```python
from build123d import *

# Parameters (mm, degrees)
SKETCH1_W           = 165.1
SKETCH1_H           = 76.2
SKETCH1_R           = 6.35
SKETCH1_R_2         = 2.50825
BOSS_EXTRUDE1_DEPTH = 6.35
CUT_EXTRUDE1_DEPTH  = 6.35
FILLET1_R           = 6.35
SKETCH3_R           = 1.778
CUT_EXTRUDE2_DEPTH  = 6.35
CIRPATTERN1_COUNT   = 8


with BuildPart() as part:
    # Sketch1 → Boss-Extrude1 (new body)
    with BuildSketch(Plane.XY):
        Rectangle(SKETCH1_W, SKETCH1_H)
        with Locations((0, -19.05)):
            Circle(SKETCH1_R, mode=Mode.SUBTRACT)
        with Locations((-75.40625, 31.75)):
            Circle(SKETCH1_R_2, mode=Mode.SUBTRACT)
        with Locations((75.40625, 31.75)):
            Circle(SKETCH1_R_2, mode=Mode.SUBTRACT)
        with Locations((75.40625, 19.05)):
            Circle(SKETCH1_R_2, mode=Mode.SUBTRACT)
        with Locations((-75.40625, 19.05)):
            Circle(SKETCH1_R_2, mode=Mode.SUBTRACT)
    extrude(amount=BOSS_EXTRUDE1_DEPTH)

    # Sketch2 → Cut-Extrude1 (cut)
    with BuildSketch(Plane(origin=(0, 0, 0), x_dir=(-1, 0, 0), z_dir=(0, 0, -1))):
        Polygon((12.7, -38.1), (82.55, 12.7), (82.55, -38.1), align=None)
        Polygon((-82.55, -38.1), (-82.55, 12.7), (-12.7, -38.1), align=None)
    extrude(amount=-CUT_EXTRUDE1_DEPTH, mode=Mode.SUBTRACT)

    # Fillet1
    fillet1_edges = [part.edges().sort_by_distance(p)[0] for p in [
        (-12.7, -38.1, 3.175),
        (-82.55, 12.7, 3.175),
        (12.7, -38.1, 3.175),
        (82.55, 12.7, 3.175),
        (-82.55, 38.1, 3.175),
        (82.55, 38.1, 3.175),
    ]]
    fillet(fillet1_edges, radius=FILLET1_R)

    # Sketch3 → Cut-Extrude2 (cut)
    with BuildSketch(Plane(origin=(0, 0, 0), x_dir=(-1, 0, 0), z_dir=(0, 0, -1))):
        with Locations((0, -9.271)):
            Circle(SKETCH3_R)
    cut_extrude2 = extrude(amount=-CUT_EXTRUDE2_DEPTH, mode=Mode.SUBTRACT)

    # CirPattern1: Cut-Extrude2 ×8 about axis
    cirpattern1_axis = Axis((0, -19.05, 0), (0, 0, 1))
    for i in range(1, CIRPATTERN1_COUNT):
        add(cut_extrude2.rotate(cirpattern1_axis, i * 360 / CIRPATTERN1_COUNT), mode=Mode.SUBTRACT)


solid = part.part
```
Verification items for the finished model (mm, model axes). Give positions to 0.01 mm unless a question says otherwise; leave off trailing zeros. Write each loop counter-clockwise with the first axis right and the second up, starting at its lowest first coordinate (ties: lowest second). Pieces come first, ordered by that corner, then holes. Notation, with made-up numbers: (20, 50.5) - (27, 50.5) arc R34 ccw to (27, 84.5) - close; hole circle Ø7 at (80, -38). An arc over 180 degrees is marked (long way). Put each result on its own line as item: value.
Q1. Section check A-A on x = 0. Record the cut outline in (y, z), and give its area (3 significant figures).
Result:
outline: (-38.1, 0) - (-30.61, 0) - (-30.61, 6.35) - (-38.1, 6.35) - close; (-27.05, 0) - (-25.4, 0) - (-25.4, 6.35) - (-27.05, 6.35) - close; (-12.7, 0) - (-11.05, 0) - (-11.05, 6.35) - (-12.7, 6.35) - close; (-7.49, 0) - (38.1, 0) - (38.1, 6.35) - (-7.49, 6.35) - close
area: 358 mm2
Q2. Mould release check, pull along Y, two halves, no side actions. Record for faces 1 (the face through (-1.38, -25.25, 3.13)), 2 (the face through (0, -38.1, 3)), 3 (the face through (-1, 9, 0)): released by +Y, released by -Y, zero draft, split by the parting line, or undercut.
Result:
face 1: undercut
face 2: released by -Y
face 3: zero draft
Q3. Depth check by flat-ended pin: P1, Ø1, axis at y = -4.5, z = 3.5, coming from the +X side; P2, Ø2, axis at x = -45, z = 2, coming from the -Y side; P3, Ø1.5, axis at y = -11, z = 4, coming from the -X side. Enter the tip coordinate at first touch or a pass-through.
Result:
P1: x = 59.59
P2: y = -15.34
P3: x = -50.99
Q4. Scan lines: probe 1 along Y at (x, z) = (0, 3.5); probe 2 along X at (y, z) = (30, 2); probe 3 along X at (y, z) = (29.5, 2.25). Record each from-to range of solid material in increasing order. Write a range as from..to.
Result:
probe 1: -38.1..-30.61, -27.05..-25.4, -12.7..-11.05, -7.49..38.1
probe 2: -82.55..-77.2, -73.61..73.61, 77.2..82.55
probe 3: -82.55..-76.51, -74.3..74.3, 76.51..82.55
Q5. Section check B-B on y = -19.05. Record the cut outline in (x, z).
Result:
outline: (-38.89, 0) - (-11.56, 0) - (-11.56, 6.35) - (-38.89, 6.35) - close; (-8, 0) - (-6.35, 0) - (-6.35, 6.35) - (-8, 6.35) - close; (6.35, 0) - (8, 0) - (8, 6.35) - (6.35, 6.35) - close; (11.56, 0) - (38.89, 0) - (38.89, 6.35) - (11.56, 6.35) - close
Q6. Section check D-D on x = -59. Record the cut outline in (y, z).
Result:
outline: (-4.43, 0) - (38.1, 0) - (38.1, 6.35) - (-4.43, 6.35) - close
Q7. Section check C-C on z = 2. Count the separate pieces of the cut face and the enclosed holes in it, and give its area (3 significant figures).
Result:
separate pieces: 1
enclosed holes: 13
area: 8,730 mm2
